Here's how the part is built. I have some questions about the finished solid (model axes, mm). A direction names the side the tool comes from. Round coordinates to 2 decimals unless told otherwise and drop trailing zeros. Write each loop counter-clockwise with the first axis right and the second up, starting at its lowest first coordinate (ties: lowest second). Pieces come first, ordered by that corner, then holes. Notation, with made-up numbers: (51, -32.5) -> (83, -32.5) arc R33 cw to (83, -2.5) -> close; hole circle Ø8 at (37, -4). An arc over 180 degrees is marked (long way). Put each result on its own line as item: value. Start each with the question number.
1. Suppose I cut it at B-B (z = 10.5). Please give me the cut outline in (x, y).
2. Suppose I cut it at C-C (y = -5.5). Please give me the cut outline in (x, z) (3 decimals), then the cut area to 3 significant figures.
3. Which directions (+Z, -Z, +X, -X, +Y, -Y) give clear straight access to the entire face, cutting with the end or side of a thin tool? Please do faces 1 (the face through (-47, -21, 34)), 2 (the face through (27, 3.209, 25)), 3 (the face through (40.467, -22, 25)).
4. Suppose I cut it at A-A (x = 46.5). Please give me the cut outline in (y, z).
5. We'd pull the mould along Z, two halves only. Please class faces 4 (the face through (55, -12.291, 25)), 5 (the face through (4, -21, -1)), 6 (the face through (-47, -21, 14)): +Z half, -Z half, draft (parallel to the pull), parting line (faces both ways), or undercut.
6. For pin 1 (4 mm diameter, centred on y = -38, z = 27.5, fed in from -X); pin 2 (5 mm diameter, centred on y = -16, z = 30, fed in from +X); pin 3 (1 mm diameter, centred on y = -30, z = 17.5, fed in from -X), each with a flat end and sliding along its axis, tell me the tip position at first contact or that it passes through.
7. I need wall thicknesses on probe 1 along X at (y, z) = (-1.25, 24); probe 2 along Y at (x, z) = (75.5, 19.5); probe 3 along X at (y, z) = (-2, 15). Which ranges of each line are inside material? Lowest first, please. Write a range as from..to.
8. Suppose I cut it at D-D (z = 19). Please give me the cut outline in (x, y), then the cut area to 3 significant figures.
```python
from build123d import *

# Parameters (mm, degrees)
SKETCH1_R                = 10
BOSS_EXTRUDE1_DEPTH      = 50
BOSS_EXTRUDE1_DEPTH_BACK = 1
SKETCH2_W                = 25
SKETCH2_H                = 20
SKETCH2_R                = 10
CUT_EXTRUDE3_DEPTH       = 50


with BuildPart() as part:
    # Sketch1 → Boss-Extrude1 (new body, two sides)
    with BuildSketch(Plane.XY) as boss_extrude1_sk:
        with BuildLine():
            Line((90.467312071, -12.290554593), (40.467312071, -12.290554593))
            Line((40.467312071, -12.290554593), (40.467312071, -31.373570191))
            Line((40.467312071, -31.373570191), (90.467312071, -31.373570191))
            Line((90.467312071, -31.373570191), (90.467312071, -46.790554593))
            Line((90.467312071, -46.790554593), (-34.532687929, -46.790554593))
            ThreePointArc((-34.532687929, -46.790554593), (-59.532687929, -21.790554593), (-34.532687929, 3.209445407))
            Line((-34.532687929, 3.209445407), (90.467312071, 3.209445407))
            Line((90.467312071, 3.209445407), (90.467312071, -12.290554593))
        make_face()
        with Locations((-34.532687929, -21.790554593)):
            Circle(SKETCH1_R, mode=Mode.SUBTRACT)
    extrude(amount=BOSS_EXTRUDE1_DEPTH)
    extrude(boss_extrude1_sk.sketch, amount=-BOSS_EXTRUDE1_DEPTH_BACK)

    # Sketch2 → Cut-Extrude3 (cut)
    with BuildSketch(Plane(origin=(0, 3.209445407, 0), x_dir=(1, 0, 0), z_dir=(0, 1, 0))):
        with Locations((-47.032687929, -24)):
            Rectangle(SKETCH2_W, SKETCH2_H)
        with Locations((65.467312071, -24)):
            Circle(SKETCH2_R)
        with BuildLine():
            ThreePointArc((90.467312071, -24.5), (83.174739834, -42.355321336), (65.467312071, -50))
            Line((65.467312071, -50), (90.467312071, -50))
            Line((90.467312071, -50), (90.467312071, -24.5))
        make_face()
        with BuildLine():
            Line((90.467312071, 1), (65.467312071, 1))
            ThreePointArc((65.467312071, 1), (83.174739834, -6.644678664), (90.467312071, -24.5))
            Line((90.467312071, -24.5), (90.467312071, 1))
        make_face()
    extrude(amount=-CUT_EXTRUDE3_DEPTH, mode=Mode.SUBTRACT)


solid = part.part
```
Verdict:
1. outline: (-34.53, -46.79) -> (86.28, -46.79) -> (86.28, -31.37) -> (40.47, -31.37) -> (40.47, -12.29) -> (86.28, -12.29) -> (86.28, 3.21) -> (-34.53, 3.21) arc R25 ccw to start; hole circle Ø20 at (-34.53, -21.79)
2. outline: (-53.496, -1) -> (65.467, -1) arc R25.505 ccw to (65.467, 50) -> (-53.496, 50) -> (-53.496, 34) -> (-34.533, 34) -> (-34.533, 14) -> (-53.496, 14) -> close; hole circle Ø20 at (65.467, 24)
2. area: 6,370 mm^2
3. face 1: -X, +Y, -Y
3. face 2: +Z, -Z, +X, -X, +Y
3. face 3: +Z, -Z, +X
4. outline: (-46.79, -1) -> (-31.37, -1) -> (-31.37, 50) -> (-46.79, 50) -> close; (-12.29, -1) -> (3.21, -1) -> (3.21, 50) -> (-12.29, 50) -> close
5. face 4: draft
5. face 5: -Z half
5. face 6: undercut
6. pin 1: stops at x = -34.53
6. pin 2: stops at x = 40.47
6. pin 3: stops at x = -29.62
7. probe 1: x = -34.53..55.47, 75.47..90.46
7. probe 2: y = -46.79..-31.37, -12.29..3.21
7. probe 3: x = -34.53..61.11, 69.83..88.63
8. outline: (-34.53, -46.79) -> (56.81, -46.79) -> (56.81, -31.37) -> (40.47, -31.37) -> (40.47, -12.29) -> (56.81, -12.29) -> (56.81, 3.21) -> (-34.53, 3.21) -> (-34.53, -11.79) arc R10 cw to (-34.53, -31.79) -> close; (74.13, -46.79) -> (89.87, -46.79) -> (89.87, -31.37) -> (74.13, -31.37) -> close; (74.13, -12.29) -> (89.87, -12.29) -> (89.87, 3.21) -> (74.13, 3.21) -> close
8. area: 4,580 mm^2
